Model file for the job. Use its own axes, mm. Face numbers are marked on the shaded views. A direction names the side the tool comes from. Coordinates: 2 decimals unless noted, no trailing zeros.
Q1. Pin check, flat tips, straight feed: P1, Ø11.5, axis at x = 21.5, z = -3, coming from the +Y side; P2, Ø1, axis at x = 2.5, z = -2, coming from the -Y side; P3, Ø6, axis at x = 12.5, z = -1, coming from the +Y side. Stop position of each tip, or through.
Q2. Which spindle directions (+Z, -Z, +X, -X, +Y, -Y) get a long thin tool onto all of the face, cutting with end or side? Do the marked faces 1, 2 and 3. Say none if no direction does.
Q3. Band-saw the part on C-C, the plane x = -20. State how many separate pieces and enclosed holes the cut face has, plus the area to 3 significant figures.
Q4. Drill centre lines: probe 1 along Z at (x, y) = (5, 16); probe 2 along X at (y, z) = (0.75, -22); probe 3 along X at (y, z) = (-4, -21). Where is each one in solid material? Low to high.
Q5. Pull direction X, two halves, no side cores. Call the marked faces 4, 5, 6 and 7: released by +X, released by -X, zero draft, split by the parting line, or undercut.
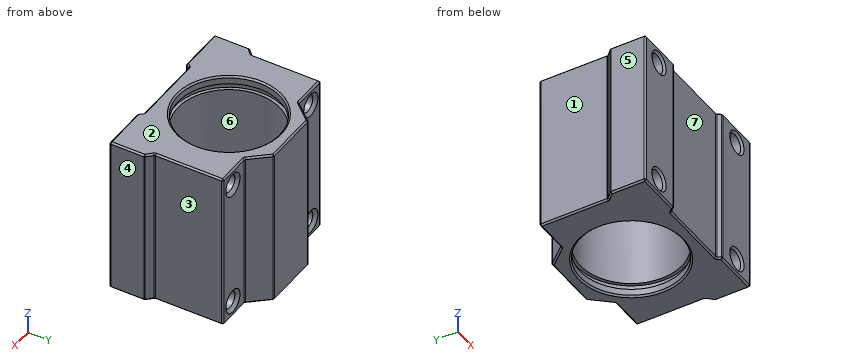
from build123d import *

# Parameters (mm, degrees)
SKETCH_1_W          = 50
SKETCH_1_H          = 40.5
EXTRUDE_1_DEPTH     = 25
SKETCH_5_R          = 2.65
CUT_EXTRUDE_2_DEPTH = 41.5
CUT_EXTRUDE_3_REACH = 52
CUT_EXTRUDE_4_DEPTH = 51
EXTRUDE_2_DEPTH     = 50
CHAMFER_1_SIZE      = 1
SKETCH_9_R          = 3
M6X12_DEPTH         = 12
FILLET_1_R          = 0.5
CHAMFER_3_SIZE      = 0.5
CUT_EXTRUDE_6_REACH = 52
SKETCH_10_R         = 16
CHAMFER_4_SIZE      = 0.5
SKETCH_11_W         = 2
SKETCH_11_H         = 17


with BuildPart() as part:
    # Эскиз1 → Бобышка-Вытянуть1 (new body, symmetric)
    with BuildSketch(Plane.XY):
        Rectangle(SKETCH_1_W, SKETCH_1_H)
    extrude(amount=EXTRUDE_1_DEPTH, both=True)

    # Эскиз5 → Вырез-Вытянуть2 (cut, through all)
    with BuildSketch(Plane(origin=(0, 20.25, 0), x_dir=(1, 0, 0), z_dir=(0, 1, 0))):
        with Locations((-20, 20)):
            Circle(SKETCH_5_R)
        with Locations((20, 20)):
            Circle(SKETCH_5_R)
        with Locations((20, -20)):
            Circle(SKETCH_5_R)
        with Locations((-20, -20)):
            Circle(SKETCH_5_R)
    extrude(amount=-CUT_EXTRUDE_2_DEPTH, mode=Mode.SUBTRACT)

    # Эскиз6 → Вырез-Вытянуть3 (cut, up to next)
    with BuildSketch(Plane.XY.offset(25), mode=Mode.PRIVATE) as cut_extrude_3_sk1:
        Polygon((-25, 14.25), (-14, 14.25), (-8.75, 20.25), (-25, 20.25), align=None)
    cut_extrude_3_tool1 = extrude(cut_extrude_3_sk1.sketch, amount=-CUT_EXTRUDE_3_REACH, mode=Mode.PRIVATE) & part.part
    add(cut_extrude_3_tool1.solids().sort_by_distance((-18.103211, 17.442661, 25))[0], mode=Mode.SUBTRACT)
    # Эскиз6 → Вырез-Вытянуть3 (cut, up to next)
    with BuildSketch(Plane.XY.offset(25), mode=Mode.PRIVATE) as cut_extrude_3_sk2:
        Polygon((25, 20.25), (25, 14.25), (14, 14.25), (8.75, 20.25), align=None)
    cut_extrude_3_tool2 = extrude(cut_extrude_3_sk2.sketch, amount=-CUT_EXTRUDE_3_REACH, mode=Mode.PRIVATE) & part.part
    add(cut_extrude_3_tool2.solids().sort_by_distance((18.103211, 17.442661, 25))[0], mode=Mode.SUBTRACT)

    # Эскиз7 → Вырез-Вытянуть4 (cut, through all)
    with BuildSketch(Plane.XY.offset(25)):
        Polygon((-12.5, -20.25), (-11.5, -18.95), (11.5, -18.95), (12.5, -20.25), align=None)
    extrude(amount=-CUT_EXTRUDE_4_DEPTH, mode=Mode.SUBTRACT)

    # Эскиз8 → Бобышка-Вытянуть2 (add)
    with BuildSketch(Plane.XY.offset(25)):
        Polygon((25, -20.25), (27, -20.25), (27, -9.25), (25, -7.25), align=None)
        Polygon((-25, -20.25), (-25, -7.25), (-27, -9.25), (-27, -20.25), align=None)
    extrude(amount=-EXTRUDE_2_DEPTH)

    # Фаска1
    chamfer_1_edges = [part.edges().sort_by_distance(p)[0] for p in [
        (-22.65, -20.25, -20),
        (17.35, -20.25, -20),
        (17.35, -20.25, 20),
        (-22.65, -20.25, 20),
        (-22.65, 14.25, 20),
        (-22.65, 14.25, -20),
        (17.35, 14.25, 20),
        (17.35, 14.25, -20),
    ]]
    chamfer(chamfer_1_edges, length=CHAMFER_1_SIZE)

    # Эскиз9 → M6x12 (cut)
    with BuildSketch(Plane.XZ.offset(20.25)):
        with Locations((-20, 20)):
            Circle(SKETCH_9_R)
        with Locations((20, 20)):
            Circle(SKETCH_9_R)
        with Locations((20, -20)):
            Circle(SKETCH_9_R)
        with Locations((-20, -20)):
            Circle(SKETCH_9_R)
    extrude(amount=-M6X12_DEPTH, mode=Mode.SUBTRACT)

    # Скругление1
    fillet_1_edges = [part.edges().sort_by_distance(p)[0] for p in [
        (-25, -7.25, 0),
        (-27, -9.25, 0),
        (-27, -20.25, 0),
        (-12.5, -20.25, 0),
        (-11.5, -18.95, 0),
        (11.5, -18.95, 0),
        (12.5, -20.25, 0),
        (27, -20.25, 0),
        (27, -9.25, 0),
        (25, -7.25, 0),
        (-25, 14.25, 0),
        (-14, 14.25, 0),
        (-8.75, 20.25, 0),
        (8.75, 20.25, 0),
        (14, 14.25, 0),
        (25, 14.25, 0),
    ]]
    fillet(fillet_1_edges, radius=FILLET_1_R)

    # Фаска3
    chamfer_3_edges = [part.edges().sort_by_distance(p)[0] for p in [
        (-25, 3.353553391, -25),
        (-25, 3.353553391, 25),
        (-26, -8.25, -25),
        (-26, -8.25, 25),
        (-19.623100374, -20.25, 25),
        (-12, -19.6, 25),
        (0, -18.95, 25),
        (12, -19.6, 25),
        (19.623100374, -20.25, 25),
        (27, -14.603553391, 25),
        (26, -8.25, 25),
        (25, 3.353553391, 25),
        (19.363442057, 14.25, 25),
        (11.375, 17.25, 25),
        (0, 20.25, 25),
        (-11.375, 17.25, 25),
        (-19.363442057, 14.25, 25),
        (-27, -14.603553391, 25),
        (24.853553391, 14.103553391, 25),
        (8.729724028, 20.205316457, 25),
        (-8.729724028, 20.205316457, 25),
        (-24.853553391, 14.103553391, 25),
        (26.961939766, -9.265765065, 25),
        (26.853553391, -20.103553391, 25),
        (12.525324868, -20.198568663, 25),
        (-12.525324868, -20.198568663, 25),
        (-26.853553391, -20.103553391, 25),
        (-26.961939766, -9.265765065, 25),
        (-27, -14.603553391, -25),
        (-12, -19.6, -25),
        (-19.623100374, -20.25, -25),
        (-19.363442057, 14.25, -25),
        (-11.375, 17.25, -25),
        (0, 20.25, -25),
        (11.375, 17.25, -25),
        (19.363442057, 14.25, -25),
        (25, 3.353553391, -25),
        (26, -8.25, -25),
        (27, -14.603553391, -25),
        (19.623100374, -20.25, -25),
        (12, -19.6, -25),
        (0, -18.95, -25),
        (24.853553391, 14.103553391, -25),
        (8.729724028, 20.205316457, -25),
        (-8.729724028, 20.205316457, -25),
        (-24.853553391, 14.103553391, -25),
        (26.961939766, -9.265765065, -25),
        (26.853553391, -20.103553391, -25),
        (12.525324868, -20.198568663, -25),
        (-12.525324868, -20.198568663, -25),
        (-26.853553391, -20.103553391, -25),
        (-26.961939766, -9.265765065, -25),
        (-25.038060234, -7.234234935, 25),
        (-25.038060234, -7.234234935, -25),
        (-11.474675132, -19.001431337, 25),
        (-11.474675132, -19.001431337, -25),
        (11.474675132, -19.001431337, 25),
        (11.474675132, -19.001431337, -25),
        (25.038060234, -7.234234935, 25),
        (25.038060234, -7.234234935, -25),
        (-14.020275972, 14.294683543, 25),
        (-14.020275972, 14.294683543, -25),
        (14.020275972, 14.294683543, 25),
        (14.020275972, 14.294683543, -25),
    ]]
    chamfer(chamfer_3_edges, length=CHAMFER_3_SIZE)

    # Эскиз10 → Вырез-Вытянуть6 (cut, up to next)
    with BuildSketch(Plane.XY.offset(25), mode=Mode.PRIVATE) as cut_extrude_6_sk1:
        with Locations((0, 0.75)):
            Circle(SKETCH_10_R)
    cut_extrude_6_tool1 = extrude(cut_extrude_6_sk1.sketch, amount=-CUT_EXTRUDE_6_REACH, mode=Mode.PRIVATE) & part.part
    add(cut_extrude_6_tool1.solids().sort_by_distance((0, 0.75, 25))[0], mode=Mode.SUBTRACT)

    # Фаска4
    chamfer_4_edges = [part.edges().sort_by_distance(p)[0] for p in [
        (-16, 0.75, -25),
        (-16, 0.75, 25),
    ]]
    chamfer(chamfer_4_edges, length=CHAMFER_4_SIZE)

    # Эскиз11 → Вырез-Повернуть1 (revolve, cut)
    with BuildSketch(Plane(origin=(0, 0, 0), x_dir=(0, 0, -1), z_dir=(1, 0, 0))):
        with Locations((-21.5, 9.25)):
            Rectangle(SKETCH_11_W, SKETCH_11_H)
        with Locations((21.5, 9.25)):
            Rectangle(SKETCH_11_W, SKETCH_11_H)
    revolve(axis=Axis((0, 0.75, 25), (0, 0, -1)), mode=Mode.SUBTRACT)


solid = part.part
Answer sheet:
1. P1: stops at y = 14.25
1. P2: stops at y = -18.95
1. P3: stops at y = 19.39
2. face 1: +Z, -Z, -X, +Y
2. face 2: +Z, +X, -X, +Y, -Y
2. face 3: +Z, -Z, +X, +Y
3. separate pieces: 3
3. enclosed holes: 0
3. area: 1,340 mm2
4. probe 1: z = -24.55 to -22.5, -20.5 to 20.5, 22.5 to 24.55
4. probe 2: x = -25 to -21.74, -18.26 to -17, 17 to 18.26, 21.74 to 25
4. probe 3: x = -25 to -22.45, -17.55 to -16.32, 16.32 to 17.55, 22.45 to 25
5. face 4: released by +X
5. face 5: released by -X
5. face 6: undercut
5. face 7: undercut
